Check sheet for the drawn part. Datum: minimum x, y, z corner. Units: mm. A direction names the side the tool comes from. Coordinates: 2 decimals unless noted, no trailing zeros. Order: outer loops, then holes, each group sorted by start corner. A loop starts at its lowest first (then second) coordinate and runs counter-clockwise, first axis right, second up. Notation, with made-up numbers: (31.25, 33) -> (43.25, 33) arc R21 ccw to (43.25, 57) -> close; hole circle Ø6 at (-7.75, 3.25). An arc over 180 degrees is marked (long way). Answer as CSV lines item,"result".
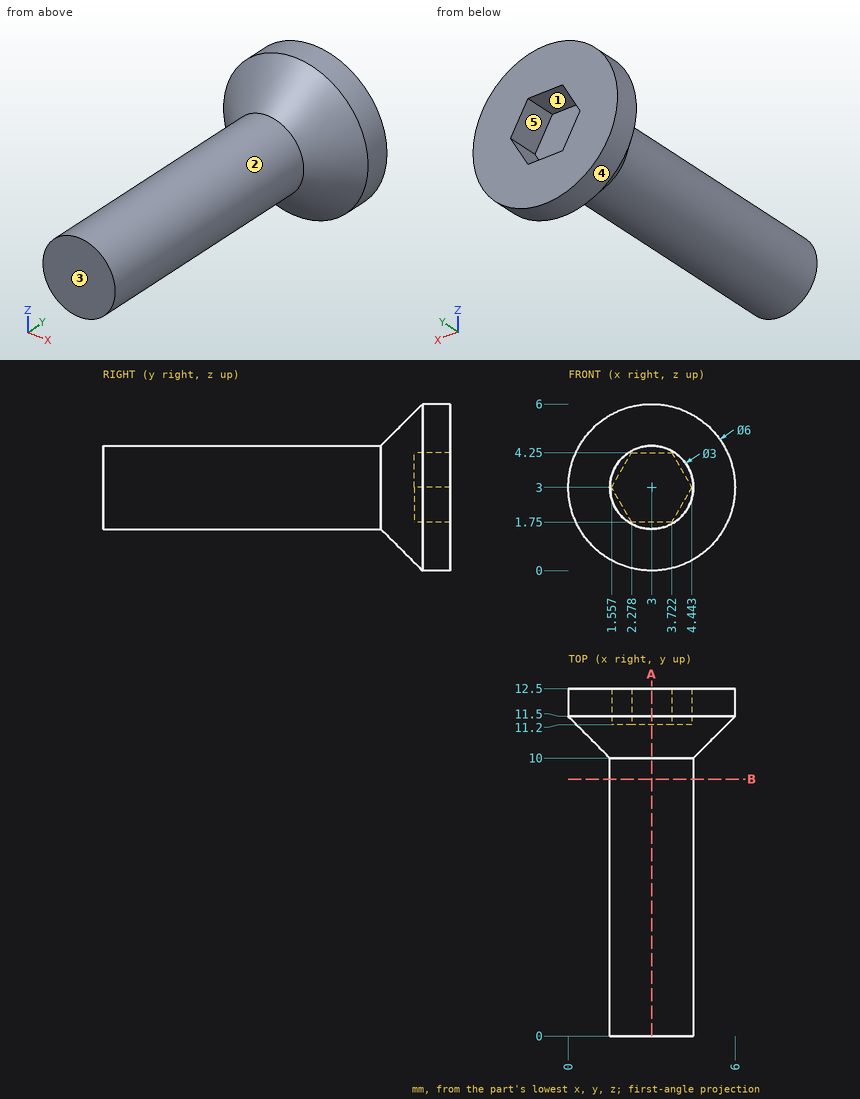
Item 1: Release check for a two-part mould opening along X. For the marked faces 1, 2 and 3 record: +X half, -X half, draft (parallel to the pull), parting line (faces both ways), or undercut.
Answer list:
face 1,"undercut"
face 2,"parting line"
face 3,"draft"
Item 2: Thickness scan on line 1 (Y direction, x = 2.6, z = 2.8); line 2 (X direction, y = 7, z = 2.9); line 3 (X direction, y = 11.75, z = 2.8). Record the ranges inside material, lowest first.
Answer list:
line 1,"0 to 11.2"
line 2,"1.5 to 4.5"
line 3,"0.01 to 1.67, 4.33 to 5.99"
Item 3: Section check B-B, the plane y = 9.25. Record the boundary of the cut face in (x, z).
Answer list:
outline,"circle Ø3 at (3, 3)"
Item 4: Depth check by flat-ended pin: pin 1 Ø1.5 at (x, z) = (3.5, 2.5) entering from -Y; pin 2 Ø0.8 at (x, z) = (3.5, 2.5) entering from +Y; pin 3 Ø1.5 at (x, z) = (4, 5.5) entering from -Y; pin 4 Ø1 at (x, y) = (1.5, 1.5) entering from +Z. Enter the tip coordinate at first touch or a pass-through.
Answer list:
pin 1,"y = 0"
pin 2,"y = 11.2"
pin 3,"y = 10.44"
pin 4,"z = 4.12"
Item 5: Section check A-A, the plane x = 3. Record the boundary of the cut face in (y, z), plus the area to 3 significant figures.
Answer list:
outline,"(0, 1.5) -> (10, 1.5) -> (11.5, 0) -> (12.5, 0) -> (12.5, 1.75) -> (11.2, 1.75) -> (11.2, 4.25) -> (12.5, 4.25) -> (12.5, 6) -> (11.5, 6) -> (10, 4.5) -> (0, 4.5) -> close"
area,"39.5 mm2"
Item 6: Tool access check on the marked faces 4 and 5. Record the directions out of +Z, -Z, +X, -X, +Y, -Y that give a thin tool (end or side, any length) a straight path to the whole face; none if there is none.
Answer list:
face 4,"+Y, -Y"
face 5,"+Y"
